Autodesk Inventor part; units mm, degrees
ref_plane "YZ Plane" through (0, 0, 0) normal (1, 0, 0) x (0, 1, 0)
ref_plane "XZ Plane" through (0, 0, 0) normal (0, 1, 0) x (-1, 0, 0)
ref_plane "XY Plane" through (0, 0, 0) normal (0, 0, 1) x (1, 0, 0)
sketch "Sketch1" plane through (0, 0, 0) normal (0, 0, 1) x (1, 0, 0)
  line L0 (-36, 53) -> (36, 53)
  line L1 (36, 53) -> (36, -53)
  line L2 (36, -53) -> (-36, -53)
  line L3 (-36, -53) -> (-36, 53)
  line L4 (-36, 53) -> (36, -53) construction
  line L5 (36, 53) -> (-36, -53) construction
  point P0 (0, 0)
  dimension "d0" = 72
  dimension "d1" = 106
extrude "Extrusion1" add sketch "Sketch1" along normal blind 3
sketch "Sketch2" plane through (0, 0, 3) normal (0, 0, 1) x (1, 0, 0)
  line L0 (-34, 53) -> (4, 53)
  line L1 (4, 53) -> (4, 41)
  line L2 (4, 41) -> (-34, 41)
  line L3 (-34, 41) -> (-34, 53)
  line L4 (36, 53) -> (-36, 53)
  line L5 (-36, 53) -> (-36, -53)
  point P0 (0, 0)
  dimension "d4" = 0
  dimension "d5" = 2
  dimension "d6" = 12
  dimension "d7" = 38
extrude "Extrusion2" cut sketch "Sketch2" against normal blind 3
sketch "Sketch3" plane through (4, 41, 3) normal (-1, 0, 0) x (0, 0, 1)
  point P0 (-3, -41)
sketch "Sketch7" plane through (-34, 41, 3) normal (0, 1, 0) x (1, 0, 0)
  line L0 (38, 3) -> (38, 0)
  line L1 (38, 3) -> (31, 3)
  line L2 (31, 3) -> (31, 0)
  line L3 (31, 0) -> (38, 0)
  line L4 (38, 0) -> (38, 3)
  point P0 (34, 3)
  dimension "d18" = 7
  dimension "d19" = 3
extrude "Extrusion5" add sketch "Sketch7" along normal blind 12
properties part number "Lid"
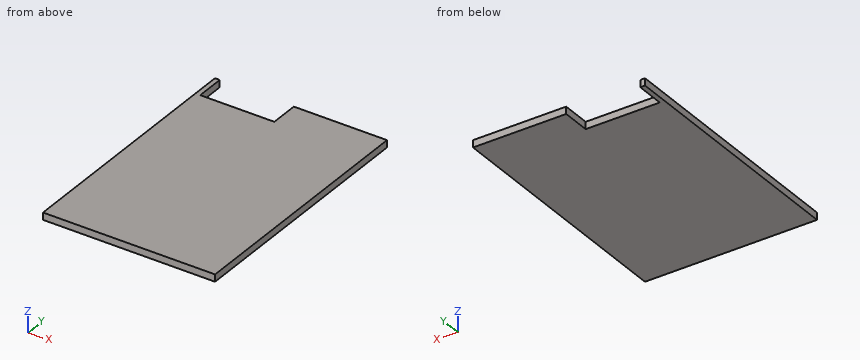
Geometry check sheet. Reference: the model listing, model coordinates, mm. Round coordinates to 2 decimals unless told otherwise and drop trailing zeros. Write each loop counter-clockwise with the first axis right and the second up, starting at its lowest first coordinate (ties: lowest second). Pieces come first, ordered by that corner, then holes.
Item 1: Section check C-C (x = -4.5). Record the boundary of the cut face in (y, z).
Determined:
outline: (-53, 0) - (41, 0) - (41, 3) - (-53, 3) - close
Item 2: Material ranges on line 1 along X through (y, z) = (47, 0.25); line 2 along Y through (x, z) = (-22, 0.95), recorded low to high.
Determined:
line 1: x = -36 to -34, -3 to 36
line 2: y = -53 to 41
Item 3: Go/stop test with a flat-tipped pin: pin 1 Ø3 at (x, y) = (-19.5, 40) entering from -Z. Record where the tip stops, or that it passes through.
Determined:
pin 1: stops at z = 0
Item 4: Section check A-A (y = 43). Record the boundary of the cut face in (x, z).
Determined:
outline: (-36, 0) - (-34, 0) - (-34, 3) - (-36, 3) - close; (-3, 0) - (36, 0) - (36, 3) - (-3, 3) - close
Item 5: Section check B-B (z = 1.1). Record the boundary of the cut face in (x, y), plus the area to 3 significant figures.
Determined:
outline: (-36, -53) - (36, -53) - (36, 53) - (-3, 53) - (-3, 41) - (-34, 41) - (-34, 53) - (-36, 53) - close
area: 7,260 mm2
